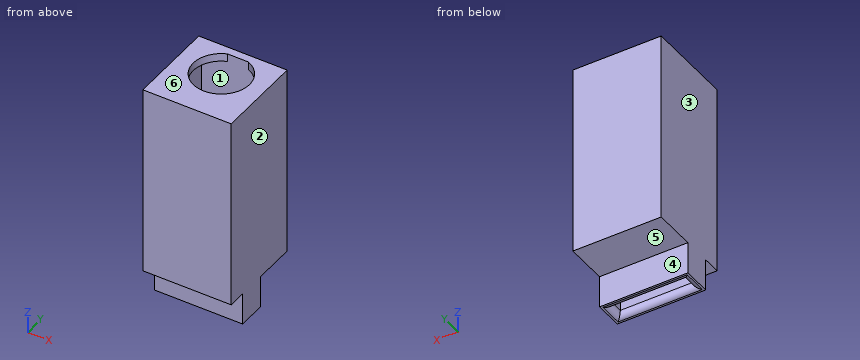
Autodesk Inventor part; units mm, degrees
ref_plane "YZ Plane" through (0, 0, 0) normal (1, 0, 0) x (0, 1, 0)
ref_plane "XZ Plane" through (0, 0, 0) normal (0, 1, 0) x (-1, 0, 0)
ref_plane "XY Plane" through (0, 0, 0) normal (0, 0, 1) x (1, 0, 0)
sketch "Sketch1" plane through (0, 0, 0) normal (0, 1, 0) x (-1, 0, 0)
  line L0 (-5.5, -12) -> (5.5, -12)
  line L1 (5.5, -12) -> (5.5, 12)
  line L2 (5.5, 12) -> (-5.5, 12)
  line L3 (-5.5, 12) -> (-5.5, -12)
  line L4 (-5.5, -12) -> (5.5, 12) construction
  line L5 (5.5, -12) -> (-5.5, 12) construction
  point P0 (0, 0)
  dimension "d0" = 11
  dimension "d1" = 24
extrude "Extrusion1" add sketch "Sketch1" along normal blind 10
shell "Shell1" thickness 1 removed faces 1 at (1.8333, 10, 4)
sketch "Sketch2" plane through (-5.5, 0, 12) normal (0, 0, 1) x (1, 0, 0)
  line L0 (0, 10) -> (11, 10)
  circle A0 centre (5.5, 6.75) radius 3.5
  point P0 (5.5, 0)
  point P1 (4.201, 10)
  point P2 (6.799, 10)
  dimension "d5" = 7
  dimension "d6" = 0.25
extrude "Extrusion2" cut sketch "Sketch2" against normal blind 9 contours L0 A0 picked at (4.7002, 5.9949)
sketch "Sketch3" plane through (0, 10, 0) normal (0, 1, 0) x (1, 0, 0)
  line L0 (1.299, -12) -> (5.5, -12)
  line L1 (5.5, -12) -> (5.5, 12)
  line L2 (5.5, 12) -> (-5.5, 12)
  line L3 (-5.5, 12) -> (-5.5, -12)
  line L4 (-5.5, -12) -> (-1.299, -12)
  line L5 (-5.5, 12) -> (5.5, 12)
  line L6 (5.5, 12) -> (5.5, -12)
  line L7 (5.5, -12) -> (-5.5, -12)
  line L8 (-5.5, -12) -> (-5.5, 12)
  point P0 (0, 0)
  point P1 (-1.299, -12)
extrude "Extrusion3" add sketch "Sketch3" along normal blind 1
sketch "Sketch4" plane through (5.5, 0, -12) normal (0, 0, -1) x (-1, 0, 0)
  line L0 (10, 1) -> (10, 10)
  line L1 (1, 1) -> (1, 10)
  line L2 (1, 3.25) -> (10, 3.25)
  line L3 (1, 1) -> (10, 1)
  line L4 (1, 4.75) -> (10, 4.75)
  line L5 (1.5, 4.75) -> (1.5, 3.25)
  line L6 (9.5, 4.75) -> (9.5, 3.25)
  point P0 (5.5, 0)
  point P1 (10, 3.25)
  dimension "d11" = 2.25
  dimension "d14" = 1.5
  dimension "d15" = 0.5
  dimension "d16" = 0.5
extrude "Extrusion4" cut sketch "Sketch4" against normal blind 10 contours L2 L6 L4 L0 | L2 L5 L4 L6 | L1 L4 L5 L2
sketch "Sketch5" plane through (5.5, 0, -12) normal (0, 0, -1) x (-1, 0, 0)
  line L0 (1, 3.25) -> (1, 4.75)
  line L1 (1, 4.75) -> (10, 4.75)
  line L2 (10, 4.75) -> (10, 3.25)
  line L3 (10, 3.25) -> (1, 3.25)
  line L4 (11, 0) -> (11, 11)
  line L5 (0, 0) -> (0, 11)
  line L6 (0, 0) -> (0, 11)
  line L7 (0, 5.75) -> (11, 5.75)
  line L8 (11, 5.75) -> (11, 2.25)
  line L9 (11, 2.25) -> (0, 2.25)
  line L10 (0, 2.25) -> (0, 5.75)
  point P0 (5.5, 0)
  point P1 (0, 2.25)
  dimension "d19" = 1
  dimension "d20" = 1
extrude "Extrusion5" add sketch "Sketch5" along normal blind 4
fillet "Fillet1" radius 0.75 4 edges at (-4.5, 4, -16) (0, 3.25, -16) (4.5, 4, -16) (0, 4.75, -16)
properties part number "carcasaXeotype_FLEX-SENSOR"
Source: CAD feature listing. Evaluate the final solid. Frame: model axes, mm. Face numbers are marked on the shaded views. A direction names the side the tool comes from. Round coordinates to 2 decimals unless told otherwise and drop trailing zeros. Loops run counter-clockwise (first coordinate to the right, second up) from the corner with the lowest first, then second, coordinate; pieces in that order, holes last. Notation, with made-up numbers: M 73.25,-11 L 109.25,-11 A26 cw 109.25,3 Z; hole C 12,43 d1. An arc over 180 degrees is marked long. Return JSON: item names as keys, results as strings. Group by question number.
1. Reachability of the marked faces 5 and 6 from +Z, -Z, +X, -X, +Y, -Y: full face, straight path, thin tool, end or side. Return the list, or none.
2. Pin query (flat end, axial travel): pin 1 (5 mm diameter, centred on x = -3.5, y = 8.5, fed in from -Z); pin 2 (1.2 mm diameter, centred on x = 2.5, z = -13.5, fed in from +Y); pin 3 (1.2 mm diameter, centred on x = 0.5, z = -13.5, fed in from -Y). Return the tip coordinate at first contact, or that it passes through.
3. Section query D-D on z = -11.5. Output: boundary loops of the cut face in (x, y).
4. Section query A-A on x = 0. Output: boundary loops of the cut face in (y, z).
5. Material intervals for line 1 along X through (y, z) = (5.75, -4.75); line 2 along Y through (x, z) = (2, -0.25); line 3 along Y through (x, z) = (-2.75, -13), sorted ascending. Write a range as from..to.
6. Section query B-B on z = -8.25. Output: boundary loops of the cut face in (x, y).
7. Mould query, pull axis X, two halves, no side actions, for the marked faces 1, 2, 3 and 4. Classes: released by +X, released by -X, zero draft, split by the parting line, or undercut.
8. Section query C-C on y = 6.75. Output: boundary loops of the cut face in (x, z), and give its area (3 significant figures).
Checks:
{
 "1": {"face 5": "-Z, +X, -X, +Y", "face 6": "+Z, +X, -X, +Y, -Y"},
 "2": {"pin 1": "stops at z = -12", "pin 2": "stops at y = 5.75", "pin 3": "stops at y = 2.25"},
 "3": {"outline": "M -5.5,0 L 5.5,0 L 5.5,11 L -5.5,11 Z; hole M -4.5,3.25 L 4.5,3.25 L 4.5,4.75 L -4.5,4.75 Z"},
 "4": {"outline": "M 0,-12 L 2.25,-12 L 2.25,-16 L 2.5,-16 A0.75 ccw 3.25,-15.25 L 3.25,-11 L 1,-11 L 1,11 L 3.25,11 L 3.25,12 L 0,12 Z; M 4.75,-15.25 A0.75 ccw 5.5,-16 L 5.75,-16 L 5.75,-12 L 11,-12 L 11,12 L 10,12 L 10,-11 L 4.75,-11 Z"},
 "5": {"line 1": "x = -5.5..-4.5, 4.5..5.5", "line 2": "y = 0..1, 10..11", "line 3": "y = 2.25..3.25, 4.75..5.75"},
 "6": {"outline": "M -5.5,0 L 5.5,0 L 5.5,11 L -5.5,11 Z; hole M -4.5,1 L 4.5,1 L 4.5,10 L -4.5,10 Z"},
 "7": {"face 1": "undercut", "face 2": "released by +X", "face 3": "released by -X", "face 4": "zero draft"},
 "8": {"outline": "M -5.5,-12 L 5.5,-12 L 5.5,12 L 3.5,12 L 3.5,11 L 4.5,11 L 4.5,-11 L -4.5,-11 L -4.5,11 L -3.5,11 L -3.5,12 L -5.5,12 Z", "area": "59.0 mm²"}
}
